Geometry: see drawing. Coordinates: mm, zero at the bounding-box minimum. Give positions to 0.01 mm unless a question says otherwise; leave off trailing zeros. Write each loop counter-clockwise with the first axis right and the second up, starting at its lowest first coordinate (ties: lowest second). Pieces come first, ordered by that corner, then holes.
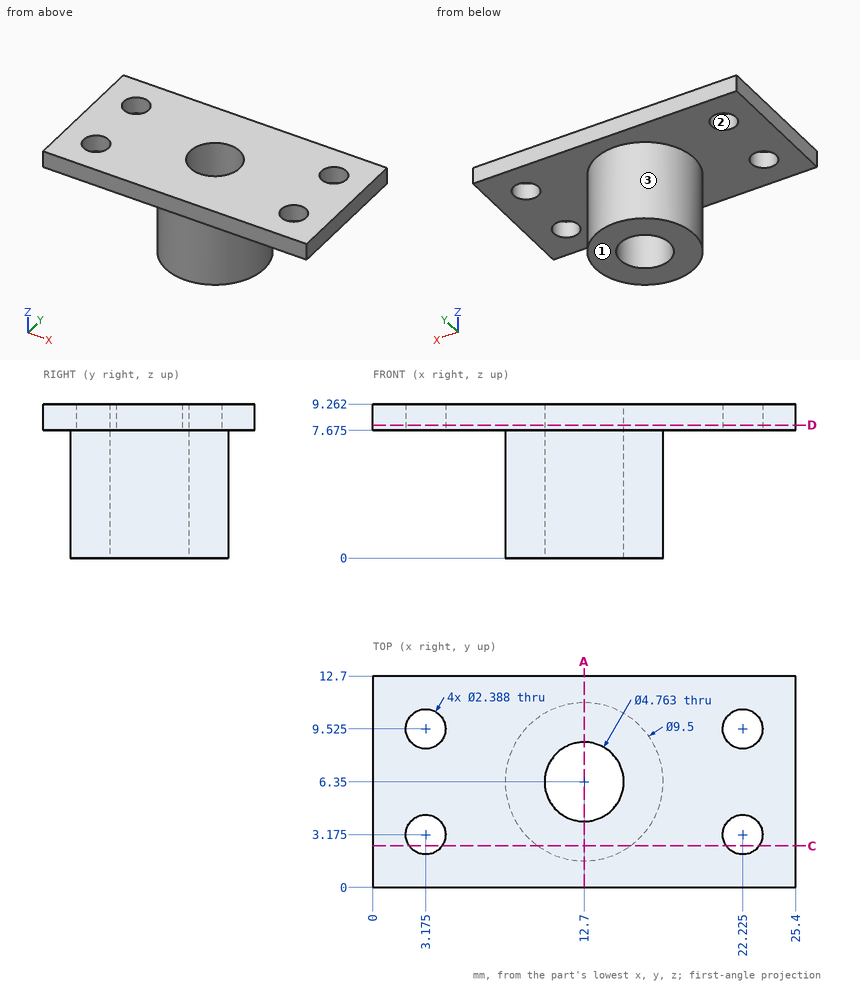
1. Section query C-C (y = 2.5). Return loops of the section in (x, z) (1 decimal).
2. Pull-direction query (X, two-part tool) for the marked faces 1, 2 and 3; classes: pulls with the +X half, pulls with the -X half, needs draft (parallel to the pull), parting line crosses it, or undercut.
3. Pin query (flat end, axial travel): P1, Ø3, axis at y = 5.5, z = 4, coming from the -X side; P2, Ø6, axis at x = 4, y = 6.5, coming from the -Z side (1 decimal); P3, Ø1.5, axis at y = 10.5, z = 3, coming from the +X side (1 decimal). Return the tip coordinate at first contact, or that it passes through.
4. Section query D-D (z = 8). Give the number of separate pieces and of enclosed holes in the cut face, plus the area to 3 significant figures.
5. Line query: probe 1 along X at (y, z) = (9.5, 8.75); probe 2 along X at (y, z) = (2.5, 8.25); probe 3 along Y at (x, z) = (12.7, 4.5). Output: solid intervals per line, ascending.
6. Section query A-A (x = 12.7). Return loops of the section in (y, z) (1 decimal).
The answers:
1. outline: (0, 7.7) - (2.2, 7.7) - (2.2, 9.3) - (0, 9.3) - close; (4.2, 7.7) - (9.9, 7.7) - (9.9, 0) - (15.5, 0) - (15.5, 7.7) - (21.2, 7.7) - (21.2, 9.3) - (4.2, 9.3) - close; (23.2, 7.7) - (25.4, 7.7) - (25.4, 9.3) - (23.2, 9.3) - close
2. face 1: needs draft
2. face 2: undercut
2. face 3: parting line crosses it
3. P1: stops at x = 7.95
3. P2: stops at z = 7.7
3. P3: stops at x = 16
4. separate pieces: 1
4. enclosed holes: 5
4. area: 287 mm2
5. probe 1: x = 0 to 1.98, 4.37 to 21.03, 23.42 to 25.4
5. probe 2: x = 0 to 2.19, 4.16 to 21.24, 23.21 to 25.4
5. probe 3: y = 1.6 to 3.97, 8.73 to 11.1
6. outline: (0, 7.7) - (1.6, 7.7) - (1.6, 0) - (4, 0) - (4, 9.3) - (0, 9.3) - close; (8.7, 0) - (11.1, 0) - (11.1, 7.7) - (12.7, 7.7) - (12.7, 9.3) - (8.7, 9.3) - close
